The listing builds one solid part. Answer for the finished solid, in the listing's coordinates (mm). A direction names the side the tool comes from. Round coordinates to 2 decimals unless told otherwise and drop trailing zeros. Order: outer loops, then holes, each group sorted by start corner. A loop starts at its lowest first (then second) coordinate and runs counter-clockwise, first axis right, second up. Notation, with made-up numbers: (-24, 24.25) - (16, 24.25) arc R25 cw to (16, 37.25) - close; hole circle Ø3 at (-17.75, -6). An arc over 180 degrees is marked (long way). Write item = value, one per line.
from build123d import *

# Parameters (mm, degrees)
F0_W     = 17
F0_H     = 3
F3_DEPTH = 3.5
F4_COUNT = 4
F5_R     = 2.99999


# Not quite as in the source:
# - a fillet or chamfer is up to 0.001 mm smaller than in the source, because OpenCascade refuses the exact size


with BuildPart() as f1:
    # F0 (on Right) → F1 (revolve)
    with BuildSketch(Plane.YZ):
        with Locations((8.5, 15)):
            Rectangle(F0_W, F0_H)
    revolve(axis=Axis((0, 4.8521989956, 0), (0, 1, 0)))



with BuildPart() as f1b:
    # F0 (on Right) → F1, piece 2 (revolve)
    with BuildSketch(Plane.YZ):
        Polygon((0, 2.2574728355), (0, 1.5), (9.8266890272, 1.5), (9.8266890272, 4.9105980434), (6.0609620996, 4.9105980434), (6.0609620996, 2.2574728355), align=None)
    revolve(axis=Axis((0, 4.8521989956, 0), (0, 1, 0)))


with BuildPart() as f1_1:
    add(f1.part)

    add(f1b.part)  # F3 merges F1b
    # F2 (on face) → F3 (join, symmetric)
    with BuildSketch(Plane.XZ.offset(-6.0609620996)):
        with BuildLine():
            Line((0, 13.3796269074), (0, 4.9105980434))
            ThreePointArc((0, 4.9105980434), (1.8559366755, 4.5463691227), (3.4365562486, 3.5077135421))
            Line((3.4365562486, 3.5077135421), (10.1425750181, 8.8311284781))
            ThreePointArc((10.1425750181, 8.8311284781), (5.6432817311, 12.3808523131), (0, 13.3796269074))
        make_face()
    extrude(amount=F3_DEPTH, both=True)

    # F4: F1 ×4 about axis
    f4_axis = Axis((0, 9.8266890272, 0), (0, 1, 0))


with BuildPart() as f1_2:
    add(f1_1.part)
    for i in range(1, F4_COUNT):
        add(f1_1.part.rotate(f4_axis, i * 360 / F4_COUNT))

    # F5 (radius 3 in the source; OpenCascade refuses exactly that, so slightly less here)
    f5_edges = [f1_2.edges().sort_by_distance(p)[0] for p in [
        (0, 0, -16.5),
        (0, 17, -16.5),
    ]]
    fillet(f5_edges, radius=F5_R)


solid = f1_2.part
Q1. Section D-D on x = -4 is taken. Count the separate pieces of the cut face and the enclosed holes in it, then the cut area to 3 significant figures.
Model answer:
separate_pieces = 3
enclosed_holes = 0
area = 190 mm^2
Q2. Flat-ended cylindrical pins translate along their axes: P1, Ø3, axis at x = 10, z = -6.5, coming from the -Y side; P2, Ø5.5, axis at y = 5.5, z = 10.5, coming from the -X side; P3, Ø1, axis at y = 3.5, z = 3.5, coming from the +X side (3 decimals). Find the tip coordinate at first contact, or state that the pin passes through.
Model answer:
P1 = 2.56
P2 = -14.57
P3 = 16.225
Q3. Section C-C on y = 13 is taken. Determine the outline of the cut face in (x, z), then the cut area to 3 significant figures.
Model answer:
outline = circle Ø33 at (0, 0); hole circle Ø27 at (0, 0)
area = 283 mm^2
Q4. Section B-B on y = 7.5 is taken. Determine the outline of the cut face in (x, z).
Model answer:
outline = circle Ø33 at (0, 0); hole (-13.38, 0) arc R11.75 cw to (-13.35, 1.99) arc R13.5 ccw to (-9.54, -9.55) arc R11.75 cw to (-10.14, -8.83) - (-3.44, -3.51) arc R4.91 cw to (-4.91, 0) - close; hole (-9.55, 9.54) arc R11.75 cw to (-8.83, 10.14) - (-3.51, 3.44) arc R4.91 cw to (0, 4.91) - (0, 13.38) arc R11.75 cw to (1.99, 13.35) arc R13.5 ccw to start; hole (-1.99, -13.35) arc R13.5 ccw to (9.55, -9.54) arc R11.75 cw to (8.83, -10.14) - (3.51, -3.44) arc R4.91 cw to (0, -4.91) - (0, -13.38) arc R11.75 cw to start; hole circle Ø3 at (0, 0); hole (3.44, 3.51) arc R4.91 cw to (4.91, 0) - (13.38, 0) arc R11.75 cw to (13.35, -1.99) arc R13.5 ccw to (9.54, 9.55) arc R11.75 cw to (10.14, 8.83) - close
Q5. For faces 1 (the face through (0, 6, -9)), 2 (the face through (9, 9.561, -4)), 3 (the face through (-4, 2.561, -9)), determine the directions among +Z, -Z, +X, -X, +Y, -Y from which every point of the face is accessible in a straight line to the end or side of a thin tool.
Model answer:
face_1 = +Y, -Y
face_2 = +Y
face_3 = -Y
Q6. Section A-A on y = 5.25 is taken. Determine the outline of the cut face in (x, z), then the cut area to 3 significant figures.
Model answer:
outline = circle Ø33 at (0, 0); circle Ø4.51 at (0, 0); hole (-13.38, 0) arc R11.75 cw to (-13.35, 1.99) arc R13.5 ccw to (-9.54, -9.55) arc R11.75 cw to (-10.14, -8.83) - (-3.44, -3.51) arc R4.91 ccw to (0, -4.91) - (0, -13.38) arc R11.75 cw to (-1.99, -13.35) arc R13.5 ccw to (9.55, -9.54) arc R11.75 cw to (8.83, -10.14) - (3.51, -3.44) arc R4.91 ccw to (4.91, 0) - (13.38, 0) arc R11.75 cw to (13.35, -1.99) arc R13.5 ccw to (9.54, 9.55) arc R11.75 cw to (10.14, 8.83) - (3.44, 3.51) arc R4.91 ccw to (0, 4.91) - (0, 13.38) arc R11.75 cw to (1.99, 13.35) arc R13.5 ccw to (-9.55, 9.54) arc R11.75 cw to (-8.83, 10.14) - (-3.51, 3.44) arc R4.91 ccw to (-4.91, 0) - close; hole circle Ø3 at (0, 0)
area = 555 mm^2
Q7. Find the intervals of material crossed by line 1 (X direction, y = 10.25, z = 0); line 2 (Z direction, x = 4, y = 6.75) (1 decimal), in increasing order. Write a range as from..to.
Model answer:
line_1 = -16.5..-13.5, 13.5..16.5
line_2 = -16..-12.9, -4.1..2.8, 4..16
